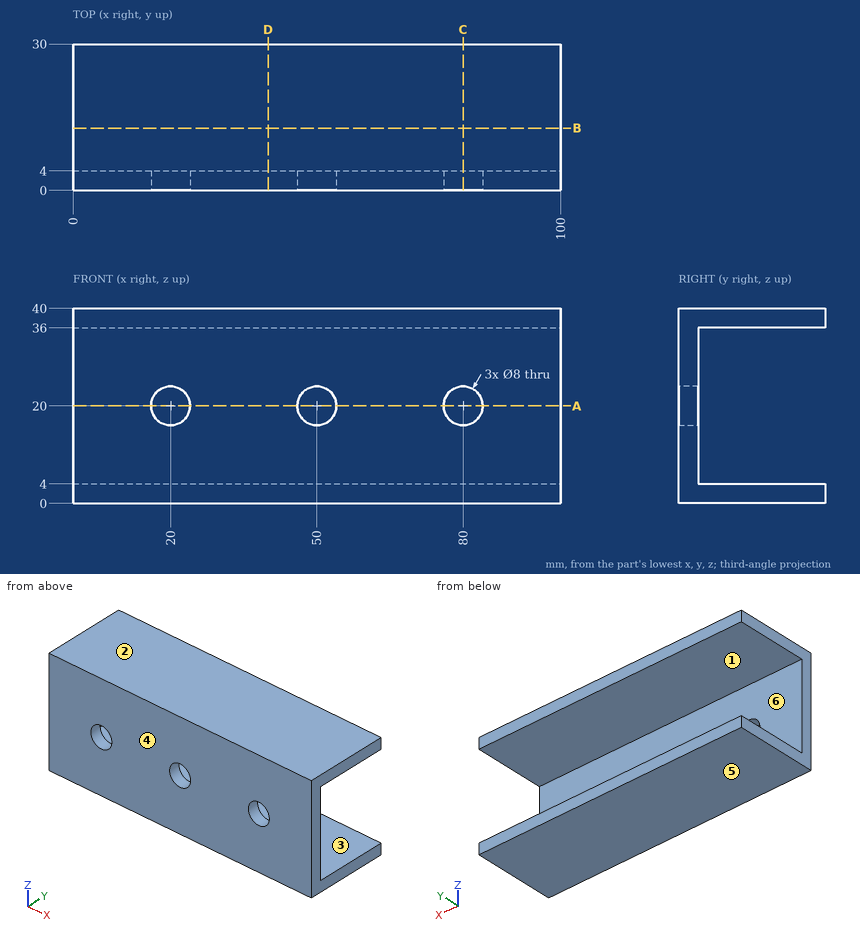
Print and shaded views of the part. All mm, measured from the part's lowest x, y and z. A direction names the side the tool comes from. Coordinates: 2 decimals unless noted, no trailing zeros. Loops run counter-clockwise (first coordinate to the right, second up) from the corner with the lowest first, then second, coordinate; pieces in that order, holes last. Notation, with made-up numbers: (-6.75, 72.5) - (46.25, 72.5) arc R25 ccw to (46.25, 103.5) - close; hole circle Ø1 at (4.25, 5). An arc over 180 degrees is marked (long way). Use one line per item in the form item = value. Start each with the question number.
1) Two-plate mould, pull along Z, no slides. Class the marked faces 1, 2, 3 and 4: +Z half, -Z half, draft (parallel to the pull), parting line (faces both ways), or undercut.
2) Flat gauge pins, fed straight in: pin 1 (1.5 mm diameter, centred on x = 67.5, y = 15.5, fed in from -Z); pin 2 (10.5 mm diameter, centred on x = 80, z = 20, fed in from +Y); pin 3 (5 mm diameter, centred on x = 50, z = 20, fed in from +Y). Where does each tip first touch, or does it go through?
3) Tool access for the marked faces 5 and 6: list every direction of +Z, -Z, +X, -X, +Y, -Y with a clear straight run to the whole face (end or side of a thin tool).
4) Band-saw the part on B-B (y = 12.75). Give the cut face in (x, z).
5) Band-saw the part on C-C (x = 80). Give the cut face in (y, z), and give its area (3 significant figures).
6) Band-saw the part on D-D (x = 40). Give the cut face in (y, z), and give its area (3 significant figures).
7) Band-saw the part on A-A (z = 20). Give the cut face in (x, y).
8) Drill centre lines: L1, parallel to X at y = 0.85, z = 20; L2, parallel to Z at x = 50, y = 1.55; L3, parallel to Z at x = 28, y = 19.5. Where is each one in solid material? Low to high. Write a range as from..to.
Check values:
q1.face_1 = undercut
q1.face_2 = +Z half
q1.face_3 = undercut
q1.face_4 = draft
q2.pin_1 = 0
q2.pin_2 = 4
q2.pin_3 = through
q3.face_5 = -Z, +X, -X, +Y, -Y
q3.face_6 = +X, -X, +Y
q4.outline = (0, 0) - (100, 0) - (100, 4) - (0, 4) - close; (0, 36) - (100, 36) - (100, 40) - (0, 40) - close
q5.outline = (0, 0) - (30, 0) - (30, 4) - (4, 4) - (4, 16) - (0, 16) - close; (0, 24) - (4, 24) - (4, 36) - (30, 36) - (30, 40) - (0, 40) - close
q5.area = 336 mm2
q6.outline = (0, 0) - (30, 0) - (30, 4) - (4, 4) - (4, 36) - (30, 36) - (30, 40) - (0, 40) - close
q6.area = 368 mm2
q7.outline = (0, 0) - (16, 0) - (16, 4) - (0, 4) - close; (24, 0) - (46, 0) - (46, 4) - (24, 4) - close; (54, 0) - (76, 0) - (76, 4) - (54, 4) - close; (84, 0) - (100, 0) - (100, 4) - (84, 4) - close
q8.L1 = 0..16, 24..46, 54..76, 84..100
q8.L2 = 0..16, 24..40
q8.L3 = 0..4, 36..40
